```python
from build123d import *

# Parameters (mm, degrees)
BOSS_EXTRUDE1_DEPTH = 15
BOSS_EXTRUDE2_DEPTH = 5
SKETCH4_W           = 200
SKETCH4_H           = 200
CUT_EXTRUDE1_DEPTH  = 1


with BuildPart() as part:
    # Sketch1 → Boss-Extrude1 (new body)
    with BuildSketch(Plane(origin=(0, 0, 0), x_dir=(1, 0, 0), z_dir=(0, 1, 0))):
        with BuildLine():
            Line((-100, 125), (100, 125))
            ThreePointArc((100, 125), (117.67766953, 117.67766953), (125, 100))
            Line((125, 100), (125, -100))
            ThreePointArc((125, -100), (117.67766953, -117.67766953), (100, -125))
            Line((100, -125), (-100, -125))
            ThreePointArc((-100, -125), (-117.67766953, -117.67766953), (-125, -100))
            Line((-125, -100), (-125, 100))
            ThreePointArc((-125, 100), (-117.67766953, 117.67766953), (-100, 125))
        make_face()
        with BuildLine():
            Line((-30.080566992, 51.914925498), (-85.040283496, 25.957462749))
            ThreePointArc((-85.040283496, 25.957462749), (-99.898608517, -2.464388108), (-80.587095233, -28.069795413))
            Line((-80.587095233, -28.069795413), (-21.174190466, -56.139590826))
            ThreePointArc((-21.174190466, -56.139590826), (59.797217034, 4.928776216), (-30.080566992, 51.914925498))
        make_face(mode=Mode.SUBTRACT)
    extrude(amount=BOSS_EXTRUDE1_DEPTH)

    # Sketch2 → Boss-Extrude2 (add)
    with BuildSketch(Plane.XZ):
        with BuildLine():
            Line((100, 125), (-100, 125))
            ThreePointArc((-100, 125), (-117.67766953, 117.67766953), (-125, 100))
            Line((-125, 100), (-125, -100))
            ThreePointArc((-125, -100), (-117.67766953, -117.67766953), (-100, -125))
            Line((-100, -125), (100, -125))
            ThreePointArc((100, -125), (117.67766953, -117.67766953), (125, -100))
            Line((125, -100), (125, 100))
            ThreePointArc((125, 100), (117.67766953, 117.67766953), (100, 125))
        make_face()
    extrude(amount=-BOSS_EXTRUDE2_DEPTH)

    # Sketch4 → Cut-Extrude1 (cut)
    with BuildSketch(Plane.XZ):
        Rectangle(SKETCH4_W, SKETCH4_H)
    extrude(amount=-CUT_EXTRUDE1_DEPTH, mode=Mode.SUBTRACT)


solid = part.part
```
Can you work these out from the model? Positions are in its coordinate system, mm. A direction names the side the tool comes from. Give positions to 0.01 mm unless a question says otherwise; leave off trailing zeros. Order: outer loops, then holes, each group sorted by start corner. A loop starts at its lowest first (then second) coordinate and runs counter-clockwise, first axis right, second up. Notation, with made-up numbers: (-12.75, 55) - (-0.75, 55) arc R20 ccw to (-0.75, 91) - close; hole circle Ø9 at (-17, 37.25). An arc over 180 degrees is marked (long way). Use a Markdown table: item, result. Add a question column.
Q1. If we section it at A-A on y = 7.5: Write out the boundary of the cut face in (x, z).
Q2. On a 3-axis mill with a long thin cutter (end or side, diameter ignored), from which of +Z, -Z, +X, -X, +Y, -Y can I reach the whole of each face in a straight line? I mean faces 5 (the flat face through (-57.176, 9.93, -39.118)), 6 (the cylindrical face through (-117.482, 7.395, 117.871)), 7 (the flat face through (-1, 1, 1)). Say none if no direction works.
Q3. I'm going to push a flat-ended pin straight in: pin 1 (12 mm diameter, centred on x = -11.5, z = -4.5, fed in from -Y). Where does the tip first touch, or does it pass through?
Q4. If we section it at B-B on z = 0: Write out the boundary of the cut face in (x, y), plus the area to 3 significant figures.
Q5. If we section it at D-D on z = 68: Write out the boundary of the cut face in (x, y).
Q6. Please list where these lines run through material, in increasing order: line 1 along X through (y, z) = (7, 0); line 2 along Z through (x, y) = (0, 9.75); line 3 along Y through (x, z) = (-95, 92).
Q7. If we section it at C-C on x = 0: Write out the boundary of the cut face in (y, z), plus the area to 3 significant figures.
Q8. If we mould it in two halves opening along Z, with no side actions, what happens to faces 1 (the cylindrical face through (-99.934, 9.93, 1.992)), 2 (the cylindrical face through (117.871, 7.395, 117.482)), 3 (the flat face through (113, 0, -2)), 4 (the cylindrical face through (-117.871, 7.395, -117.482))? For each: released by +Z, released by -Z, zero draft, split by the parting line, or undercut.
Answers follow:
| question | item | result |
|---|---|---|
| 1 | outline | (-125, -100) arc R25 ccw to (-100, -125) - (100, -125) arc R25 ccw to (125, -100) - (125, 100) arc R25 ccw to (100, 125) - (-100, 125) arc R25 ccw to (-125, 100) - close; hole (-85.04, -25.96) - (-30.08, -51.91) arc R60 ccw (long way) to (-21.17, 56.14) - (-80.59, 28.07) arc R30 ccw to start |
| 2 | face 5 | +Y |
| 2 | face 6 | +Z, -X, +Y, -Y |
| 2 | face 7 | -Y |
| 3 | pin 1 | stops at y = 1 |
| 4 | outline | (-125, 0) - (-100, 0) - (-100, 1) - (100, 1) - (100, 0) - (125, 0) - (125, 15) - (60, 15) - (60, 5) - (-100, 5) - (-100, 15) - (-125, 15) - close |
| 4 | area | 1,950 mm^2 |
| 5 | outline | (-125, 0) - (-100, 0) - (-100, 1) - (100, 1) - (100, 0) - (125, 0) - (125, 15) - (-125, 15) - close |
| 6 | line 1 | x = -125 to -100, 60 to 125 |
| 6 | line 2 | z = -125 to -60, 60 to 125 |
| 6 | line 3 | y = 1 to 15 |
| 7 | outline | (0, -125) - (15, -125) - (15, -60) - (5, -60) - (5, 60) - (15, 60) - (15, 125) - (0, 125) - (0, 100) - (1, 100) - (1, -100) - (0, -100) - close |
| 7 | area | 2,350 mm^2 |
| 8 | face 1 | undercut |
| 8 | face 2 | released by +Z |
| 8 | face 3 | zero draft |
| 8 | face 4 | released by -Z |
